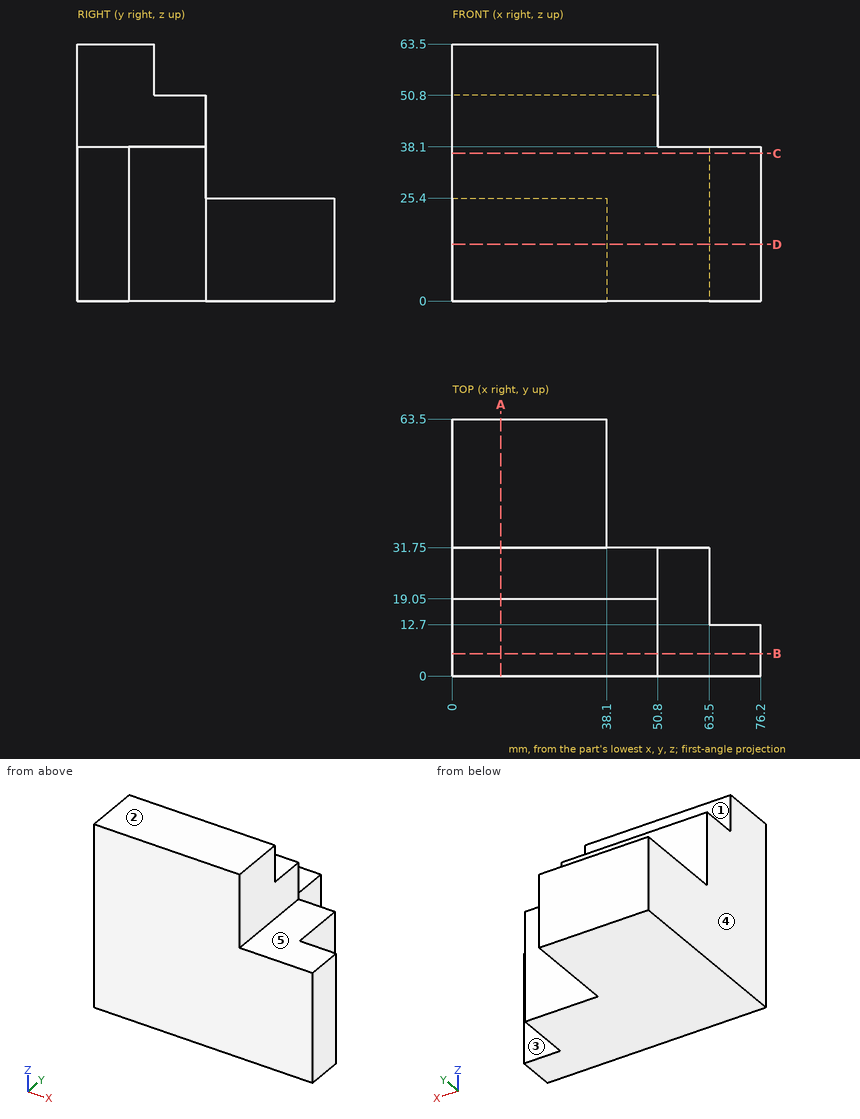
Geometry: see drawing. Coordinates: mm, zero at the bounding-box minimum. A direction names the side the tool comes from. Give positions to 0.01 mm unless a question says otherwise; leave off trailing zeros. Loops run counter-clockwise (first coordinate to the right, second up) from the corner with the lowest first, then second, coordinate; pieces in that order, holes last. Notation, with made-up numbers: (-24.5, 64.5) -> (-16.5, 64.5) arc R26 cw to (-16.5, 94.5) -> close; hole circle Ø4 at (41, -9.5). An arc over 180 degrees is marked (long way). Put each result on its own line as item: value.
1. Cut plane A-A (x = 12). Return the cut outline in (y, z), plus the area to 3 significant figures.
Taken from the geometry:
outline: (0, 0) -> (63.5, 0) -> (63.5, 25.4) -> (31.75, 25.4) -> (31.75, 50.8) -> (19.05, 50.8) -> (19.05, 63.5) -> (0, 63.5) -> close
area: 2,660 mm2
2. Cut plane D-D (z = 14). Return the cut outline in (x, y), plus the area to 3 significant figures.
Taken from the geometry:
outline: (0, 0) -> (76.2, 0) -> (76.2, 12.7) -> (63.5, 12.7) -> (63.5, 31.75) -> (38.1, 31.75) -> (38.1, 63.5) -> (0, 63.5) -> close
area: 3,390 mm2
3. Cut plane B-B (y = 5.5). Return the cut outline in (x, z), plus the area to 3 significant figures.
Taken from the geometry:
outline: (0, 0) -> (76.2, 0) -> (76.2, 38.1) -> (50.8, 38.1) -> (50.8, 63.5) -> (0, 63.5) -> close
area: 4,190 mm2
4. Ray query, line 1 along X through (y, z) = (26, 32); line 2 along X through (y, z) = (32.5, 10.5); line 3 along Y through (x, z) = (4, 41). Return the intervals inside material, ascending. Write a range as [from, to].
Taken from the geometry:
line 1: x = [0, 63.5]
line 2: x = [0, 38.1]
line 3: y = [0, 31.75]
5. Set-up query: the marked faces 1, 2, 3, 4 and 5. Return all of +Z, -Z, +X, -X, +Y, -Y with unobstructed straight access to the full face (end or side cutting, diameter ignored); none if empty.
Taken from the geometry:
face 1: +Z, +X, -X, +Y
face 2: +Z, +X, -X, +Y, -Y
face 3: +Z, -Z, +X, +Y
face 4: +Z, -Z, -X, +Y, -Y
face 5: +Z, +X, +Y, -Y
6. Cut plane C-C (z = 36.5). Return the cut outline in (x, y).
Taken from the geometry:
outline: (0, 0) -> (76.2, 0) -> (76.2, 12.7) -> (63.5, 12.7) -> (63.5, 31.75) -> (0, 31.75) -> close
7. Pin query (flat end, axial travel): P1, Ø9.5, axis at y = 19, z = 16, coming from the +X side; P2, Ø5, axis at x = 64.5, z = 8.5, coming from the +Y side; P3, Ø12.5, axis at x = 67, y = 14, coming from the +Z side; P4, Ø10, axis at x = 56, z = 46, coming from the -Y side. Return the tip coordinate at first contact, or that it passes through.
Taken from the geometry:
P1: stops at x = 63.5
P2: stops at y = 31.75
P3: stops at z = 38.1
P4: passes through
